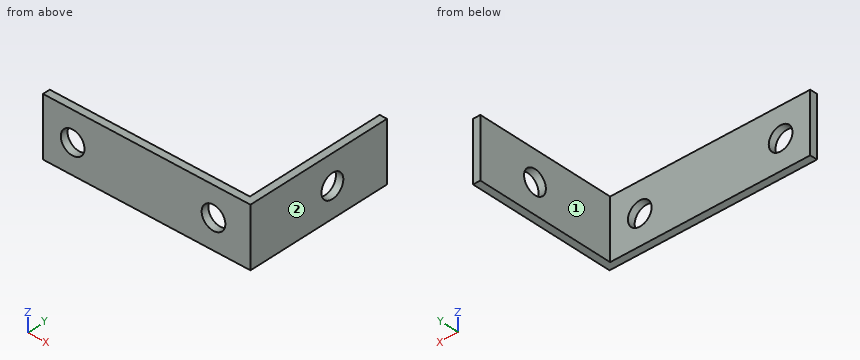
```python
from build123d import *

# Parameters (mm, degrees)
BOSS_EXTRUDE1_DEPTH = 12.7
SKETCH2_R           = 2.54
CUT_EXTRUDE1_DEPTH  = 2.5748
SKETCH3_R           = 2.54
CUT_EXTRUDE2_DEPTH  = 2.5748


with BuildPart() as part:
    # Sketch1 → Boss-Extrude1 (new body)
    with BuildSketch(Plane.XY):
        Polygon((0, 0), (44.45, 0), (44.45, 31.75), (42.8752, 31.75), (42.8752, 1.5748), (0, 1.5748), align=None)
    extrude(amount=BOSS_EXTRUDE1_DEPTH)

    # Sketch2 → Cut-Extrude1 (cut, through all)
    with BuildSketch(Plane.ZY.offset(-42.8752)):
        with Locations((6.35, 19.05)):
            Circle(SKETCH2_R)
    extrude(amount=-CUT_EXTRUDE1_DEPTH, mode=Mode.SUBTRACT)

    # Sketch3 → Cut-Extrude2 (cut, through all)
    with BuildSketch(Plane(origin=(0, 1.5748, 0), x_dir=(1, 0, 0), z_dir=(0, 1, 0))):
        with Locations((6.35, -6.35)):
            Circle(SKETCH3_R)
        with Locations((36.5252, -6.35)):
            Circle(SKETCH3_R)
    extrude(amount=-CUT_EXTRUDE2_DEPTH, mode=Mode.SUBTRACT)


solid = part.part
```
Check sheet for the modelled part. Datum: model origin and axes. Units: mm. Face numbers are marked on the shaded views. A direction names the side the tool comes from. Give positions to 0.01 mm unless a question says otherwise; leave off trailing zeros. Write each loop counter-clockwise with the first axis right and the second up, starting at its lowest first coordinate (ties: lowest second). Pieces come first, ordered by that corner, then holes. Notation, with made-up numbers: (-21.5, 27) -> (11.5, 27) arc R22 ccw to (11.5, 44) -> close; hole circle Ø6 at (81, -25). An arc over 180 degrees is marked (long way). Use CSV: the item, a comma, the result in double quotes. Start each with the question number.
Q1. Depth check by flat-ended pin: P1, Ø10, axis at x = 13.5, y = 7.5, coming from the -Z side; P2, Ø6.5, axis at y = 20.5, z = 3.5, coming from the -X side; P3, Ø2, axis at x = 6.5, z = 8, coming from the +Y side. Enter the tip coordinate at first touch or a pass-through.
Q2. Cross-section at D-D on z = 2. Enter the section's corners in (x, y).
Q3. Tool access check on the marked faces 1 and 2. Record the directions out of +Z, -Z, +X, -X, +Y, -Y that give a thin tool (end or side, any length) a straight path to the whole face; none if there is none.
Q4. Cross-section at B-B on y = 19.05. Enter the section's corners in (x, z), and give its area (3 significant figures).
Q5. Cross-section at A-A on x = 6.35. Enter the section's corners in (y, z), and give its area (3 significant figures).
Q6. Cross-section at C-C on z = 6.35. Enter the section's corners in (x, y).
Q7. Scan lines: line 1 along X through (y, z) = (0.6, 6.35); line 2 along Y through (x, z) = (43.7, 6.35); line 3 along Z through (x, y) = (6.35, 0.45). Record each from-to range of solid material in increasing order.
Working result:
1,P1,"passes through"
1,P2,"stops at x = 42.88"
1,P3,"stops at y = 1.57"
2,outline,"(0, 0) -> (44.45, 0) -> (44.45, 31.75) -> (42.88, 31.75) -> (42.88, 1.57) -> (0, 1.57) -> close"
3,face 1,"+Z, -Z, -X, +Y"
3,face 2,"+Z, -Z, +X, +Y, -Y"
4,outline,"(42.88, 0) -> (44.45, 0) -> (44.45, 3.81) -> (42.88, 3.81) -> close; (42.88, 8.89) -> (44.45, 8.89) -> (44.45, 12.7) -> (42.88, 12.7) -> close"
4,area,"12.0 mm^2"
5,outline,"(0, 0) -> (1.57, 0) -> (1.57, 3.81) -> (0, 3.81) -> close; (0, 8.89) -> (1.57, 8.89) -> (1.57, 12.7) -> (0, 12.7) -> close"
5,area,"12.0 mm^2"
6,outline,"(0, 0) -> (3.81, 0) -> (3.81, 1.57) -> (0, 1.57) -> close; (8.89, 0) -> (33.99, 0) -> (33.99, 1.57) -> (8.89, 1.57) -> close; (39.07, 0) -> (44.45, 0) -> (44.45, 16.51) -> (42.88, 16.51) -> (42.88, 1.57) -> (39.07, 1.57) -> close; (42.88, 21.59) -> (44.45, 21.59) -> (44.45, 31.75) -> (42.88, 31.75) -> close"
7,line 1,"x = 0 to 3.81, 8.89 to 33.99, 39.07 to 44.45"
7,line 2,"y = 0 to 16.51, 21.59 to 31.75"
7,line 3,"z = 0 to 3.81, 8.89 to 12.7"
